Autodesk Inventor part; units mm, degrees
ref_plane "YZ Plane" through (0, 0, 0) normal (1, 0, 0) x (0, 1, 0)
ref_plane "XZ Plane" through (0, 0, 0) normal (0, 1, 0) x (-1, 0, 0)
ref_plane "XY Plane" through (0, 0, 0) normal (0, 0, 1) x (1, 0, 0)
sketch "Sketch1" plane through (0, 0, 0) normal (0, 0, 1) x (1, 0, 0)
  line L0 (-5.1962, 0) -> (-2.5981, 4.5)
  line L1 (-2.5981, 4.5) -> (2.5981, 4.5)
  line L2 (2.5981, 4.5) -> (5.1962, 0)
  line L3 (5.1962, 0) -> (2.5981, -4.5)
  line L4 (2.5981, -4.5) -> (-2.5981, -4.5)
  line L5 (-2.5981, -4.5) -> (-5.1962, 0)
  point P0 (0, 0)
  point P1 (0, 0)
  dimension "d0" = 9
extrude "Extrusion1" add sketch "Sketch1" along normal blind 7
sketch "Sketch2" plane through (0, 0, 7) normal (0, 0, 1) x (1, 0, 0)
  circle A0 centre (0, 0) radius 3
  dimension "d3" = 6
extrude "Extrusion2" add sketch "Sketch2" along normal blind 2
sketch "Sketch3" plane through (0, 0, 0) normal (0, 0, -1) x (-1, 0, 0)
  circle A0 centre (0, 0) radius 3
  dimension "d6" = 6
extrude "Extrusion3" add sketch "Sketch3" along normal blind 5
sketch "Sketch4" plane through (0, 0, 9) normal (0, 0, 1) x (1, 0, 0)
  circle A0 centre (0, 0) radius 1.585
  dimension "d9" = 3.17
extrude "Extrusion4" cut sketch "Sketch4" against normal through all
thread "Thread1"
thread "Thread2"
properties part number "mainBody" material "Nickel-Copper Alloy 400"
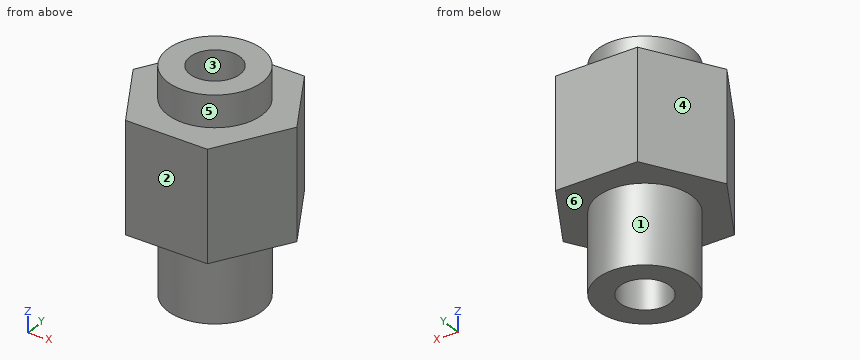
The model under review builds one solid part; all positions refer to its coordinate system, in mm. Face numbers are marked on the shaded views. A direction names the side the tool comes from. Give positions to 0.01 mm unless a question says otherwise; leave off trailing zeros. Write each loop counter-clockwise with the first axis right and the second up, starting at its lowest first coordinate (ties: lowest second). Pieces come first, ordered by that corner, then holes.
(1) Consider section B-B, the plane z = 6.5. Give the boundary of the cut face in (x, y) (3 decimals), and give its area (3 significant figures).
(2) To check wall thickness, follow L1, parallel to Y at x = 0, z = 6 (3 decimals); L2, parallel to Z at x = 4.5, y = 1; L3, parallel to X at y = 1, z = 1.5. State the ranges of each line that lie inside material, in increasing order.
(3) The part is to be moulded in two halves that separate along Y. For the marked faces 1, 2 and 3, say which applies: released by +Y, released by -Y, zero draft, split by the parting line, or undercut.
(4) Consider section D-D, the plane x = -1.75. Give the boundary of the cut face in (y, z).
(5) Consider section A-A, the plane x = 0. Give the boundary of the cut face in (y, z) (3 decimals).
(6) Tool access review of the marked faces 4, 5 and 6: name each direction out of +Z, -Z, +X, -X, +Y, -Y from which nothing blocks a thin tool from reaching the whole face with its end or side.
(7) For P1, Ø1, axis at y = 3.5, z = 1, coming from the -X side; P2, Ø1, axis at x = 4, z = -2.5, coming from the +Y side; P3, Ø1, axis at x = 3.5, z = 7, coming from the -Y side, all flat-tipped, find the tip position at first contact; note any pin that passes through.
(8) Consider section C-C, the plane y = -0.5. Give the boundary of the cut face in (x, z).
Returned:
1. outline: (-5.196, 0) - (-2.598, -4.5) - (2.598, -4.5) - (5.196, 0) - (2.598, 4.5) - (-2.598, 4.5) - close; hole circle Ø3.17 at (0, 0)
1. area: 62.3 mm2
2. L1: y = -4.5 to -1.585, 1.585 to 4.5
2. L2: z = 0 to 7
2. L3: x = -4.62 to -1.23, 1.23 to 4.62
3. face 1: split by the parting line
3. face 2: released by -Y
3. face 3: undercut
4. outline: (-4.5, 0) - (-2.44, 0) - (-2.44, -5) - (2.44, -5) - (2.44, 0) - (4.5, 0) - (4.5, 7) - (2.44, 7) - (2.44, 9) - (-2.44, 9) - (-2.44, 7) - (-4.5, 7) - close
5. outline: (-4.5, 0) - (-3, 0) - (-3, -5) - (-1.585, -5) - (-1.585, 9) - (-3, 9) - (-3, 7) - (-4.5, 7) - close; (1.585, -5) - (3, -5) - (3, 0) - (4.5, 0) - (4.5, 7) - (3, 7) - (3, 9) - (1.585, 9) - close
6. face 4: +Z, -Z, -X, +Y
6. face 5: +Z
6. face 6: -Z
7. P1: stops at x = -3.46
7. P2: passes through
7. P3: stops at y = -3.8
8. outline: (-4.91, 0) - (-2.96, 0) - (-2.96, -5) - (-1.5, -5) - (-1.5, 9) - (-2.96, 9) - (-2.96, 7) - (-4.91, 7) - close; (1.5, -5) - (2.96, -5) - (2.96, 0) - (4.91, 0) - (4.91, 7) - (2.96, 7) - (2.96, 9) - (1.5, 9) - close
